```python
from build123d import *

# Parameters (mm, degrees)
SKETCH_1_W                = 60
SKETCH_1_H                = 60
EXTRUDE_1_DEPTH           = 10
HOLE_WIZARD_1_D           = 8.5
HOLE_WIZARD_1_DEPTH       = 20
HOLE_WIZARD_2_D           = 8
HOLE_WIZARD_2_CSINK_D     = 8.2
HOLE_WIZARD_2_CSINK_ANGLE = 45
HOLE_WIZARD_3_D           = 3.2
SKETCH_8_R                = 4.6
SKETCH_8_R_2              = 4.1
EXTRUDE_2_DEPTH           = 10
EXTRUDE_START             = 4
SKETCH_10_R               = 2.55
SKETCH_10_R_2             = 1.6
EXTRUDE_4_DEPTH           = 4
SKETCH_11_W               = 60
SKETCH_11_H               = 80
EXTRUDE_5_DEPTH           = 11.75
SKETCH_12_W               = 10
SKETCH_12_H               = 20
CUT_EXTRUDE_3_DEPTH       = 90.850222593
SKETCH_13_W               = 40
SKETCH_13_H               = 20
CUT_EXTRUDE_4_DEPTH       = 4.25
HOLE_WIZARD_4_D           = 3.3
CHAMFER_1_SIZE            = 2


with BuildPart() as part:
    # 草图1 → 凸台-拉伸1 (new body)
    with BuildSketch(Plane.XY):
        Rectangle(SKETCH_1_W, SKETCH_1_H)
    extrude(amount=EXTRUDE_1_DEPTH)

    # 孔1
    with Locations(Plane.XY.offset(10)):
        with Locations((0, 0)):
            Hole(HOLE_WIZARD_1_D / 2, depth=HOLE_WIZARD_1_DEPTH)

    # 孔2 (through all)
    with Locations(Plane.XY.offset(10)):
        with Locations((20, 0), (-20, 0)):
            CounterSinkHole(HOLE_WIZARD_2_D / 2, HOLE_WIZARD_2_CSINK_D / 2, counter_sink_angle=HOLE_WIZARD_2_CSINK_ANGLE)

    # 孔3 (through all)
    with Locations(Plane(origin=(0, 0, 0), x_dir=(-1, 0, 0), z_dir=(0, 0, -1))):
        with Locations((0, 18.25), (0, -18.25)):
            Hole(HOLE_WIZARD_3_D / 2)

    # 草图8 → 凸台-拉伸2 (add)
    with BuildSketch(Plane.XY.offset(10)):
        with Locations(Location((-20, 0, 0), (0, 0, 180))):
            Circle(SKETCH_8_R)
        with Locations((-20, 0)):
            Circle(SKETCH_8_R_2, mode=Mode.SUBTRACT)
    extrude_2 = extrude(amount=EXTRUDE_2_DEPTH)

    # 镜向1: 凸台-拉伸2 across plane
    add(extrude_2.mirror(Plane(origin=(0, 0, 0), x_dir=(0, 0, 1), z_dir=(1, 0, 0))))

    # 草图10 → 凸台-拉伸4 (add)
    with BuildSketch(Plane.XY.offset(10).offset(EXTRUDE_START)):
        with Locations(Location((0, 18.25, 0), (0, 0, 180))):
            Circle(SKETCH_10_R)
        with Locations(Location((0, 18.25, 0), (0, 0, 180))):
            Circle(SKETCH_10_R_2, mode=Mode.SUBTRACT)
    extrude_4 = extrude(amount=-EXTRUDE_4_DEPTH)

    # 镜向4: 凸台-拉伸4 across plane
    add(extrude_4.mirror(Plane.ZX))

    # 草图11 → 凸台-拉伸5 (add)
    with BuildSketch(Plane.XZ.offset(30)):
        with Locations((0, 5)):
            Rectangle(SKETCH_11_W, SKETCH_11_H)
    extrude(amount=EXTRUDE_5_DEPTH)

    # 草图12 → 切除-拉伸3 (cut, through all)
    with BuildSketch(Plane.XZ.offset(41.75)):
        with Locations((-25, -25)):
            Rectangle(SKETCH_12_W, SKETCH_12_H)
        with Locations((25, -25)):
            Rectangle(SKETCH_12_W, SKETCH_12_H)
    extrude(amount=-CUT_EXTRUDE_3_DEPTH, mode=Mode.SUBTRACT)

    # 草图13 → 切除-拉伸4 (cut)
    with BuildSketch(Plane(origin=(0, -30, 0), x_dir=(1, 0, 0), z_dir=(0, 1, 0))):
        with Locations((0, 25)):
            Rectangle(SKETCH_13_W, SKETCH_13_H)
    extrude(amount=-CUT_EXTRUDE_4_DEPTH, mode=Mode.SUBTRACT)

    # 孔4 (through all)
    with Locations(Plane(origin=(0, -41.75, 0), x_dir=(-1, 0, 0), z_dir=(0, -1, 0))):
        with Locations((-10, 25), (10, 25)):
            Hole(HOLE_WIZARD_4_D / 2)

    # 倒角1
    chamfer_1_edges = [part.edges().sort_by_distance(p)[0] for p in [
        (-30, 30, 5),
        (30, 30, 5),
    ]]
    chamfer(chamfer_1_edges, length=CHAMFER_1_SIZE)


solid = part.part
```
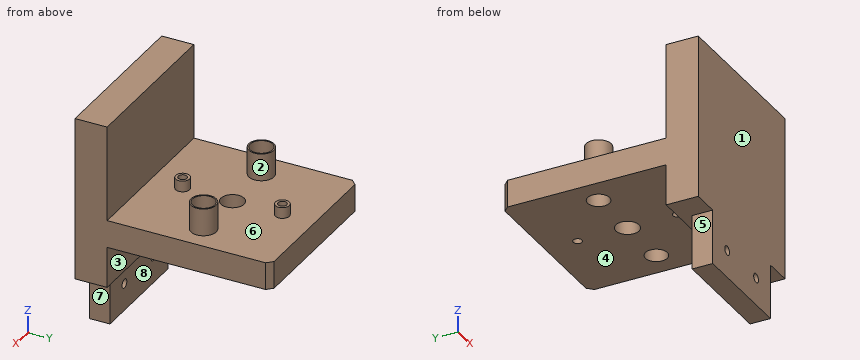
Build history of the part. All positions in model axes, mm. Face numbers are marked on the shaded views. A direction names the side the tool comes from. Give positions to 0.01 mm unless a question says otherwise; leave off trailing zeros. Order: outer loops, then holes, each group sorted by start corner. A loop starts at its lowest first (then second) coordinate and runs counter-clockwise, first axis right, second up. Notation, with made-up numbers: M -17.75,-37 L 9.25,-37 A33 ccw 9.25,-3 Z; hole C 29,51 d3. An arc over 180 degrees is marked long. Write item = value, one per line. Start each with the question number.
(1) Which spindle directions (+Z, -Z, +X, -X, +Y, -Y) get a long thin tool onto all of the face, cutting with end or side? Do the marked faces 5, 6, 7 and 8. Say none if no direction does.
(2) Slice it at D-D on y = -18.25. Write the cut outline in (x, z), plus the area to 3 significant figures.
(3) Pin check, flat tips, straight feed: pin 1 Ø5 at (x, y) = (-20, 0) entering from +Z; pin 2 Ø4 at (x, z) = (9, -20.5) entering from +Y; pin 3 Ø10 at (y, z) = (-30.5, -22.5) entering from +X; pin 4 Ø11 at (x, y) = (0, 0) entering from -Z. Stop position of each tip, or through.
(4) Two-plate mould, pull along Y, no slides. Class the marked faces 1, 2, 3 and 4: released by +Y, released by -Y, zero draft, split by the parting line, or undercut.
(5) Probe L1, parallel to Y at x = 0, z = 2.25; L2, parallel to Y at x = -20, z = 4; L3, parallel to X at y = 18, z = 12. List the from-to ranges inside material, lowest first. Write a range as [from, to].
(6) Slice it at B-B on y = -35.5. Write the cut outline in (x, z), plus the area to 3 significant figures.
(7) Slice it at C-C on x = -10. Write the cut outline in (y, z).
(8) Slice it at A-A on z = -25. Write the cut outline in (x, y).
Responses:
q1.face_5 = -Z, -X, +Y, -Y
q1.face_6 = +Z
q1.face_7 = -Z, +X, +Y, -Y
q1.face_8 = -Z, +X, -X, +Y
q2.outline = M -30,0 L -1.6,0 L -1.6,14 L -2.55,14 L -2.55,10 L -30,10 Z; M 1.6,0 L 30,0 L 30,10 L 2.55,10 L 2.55,14 L 1.6,14 Z
q2.area = 576 mm2
q3.pin_1 = through
q3.pin_2 = -34.25
q3.pin_3 = 20
q3.pin_4 = 0
q4.face_1 = released by -Y
q4.face_2 = undercut
q4.face_3 = released by +Y
q4.face_4 = zero draft
q5.L1 = [-41.75, -19.85], [-16.65, -4.25], [4.25, 16.65], [19.85, 30]
q5.L2 = [-41.75, -4], [4, 30]
q5.L3 = [-2.54, -1.58], [1.58, 2.54]
q6.outline = M -30,-15 L -20,-15 L -20,-35 L 20,-35 L 20,-15 L 30,-15 L 30,45 L -30,45 Z; hole C -10,-25 d3.3; hole C 10,-25 d3.3
q6.area = 4,380 mm2
q7.outline = M -41.75,-35 L -34.25,-35 L -34.25,-26.65 L -41.75,-26.65 Z; M -41.75,-23.35 L -34.25,-23.35 L -34.25,-15 L -30,-15 L -30,0 L 30,0 L 30,10 L -30,10 L -30,45 L -41.75,45 Z
q8.outline = M -20,-41.75 L -11.65,-41.75 L -11.65,-34.25 L -20,-34.25 Z; M -8.35,-41.75 L 8.35,-41.75 L 8.35,-34.25 L -8.35,-34.25 Z; M 11.65,-41.75 L 20,-41.75 L 20,-34.25 L 11.65,-34.25 Z
